```python
from build123d import *

# Parameters (mm, degrees)
SKETCH1_W               = 52
SKETCH1_H               = 25
BOSS_EXTRUDE1_DEPTH     = 24.18
SKETCH4_W               = 48
SKETCH4_H               = 21.11598097
CUT_EXTRUDE1_DEPTH      = 25
SKETCH6_R               = 1
SKETCH6_R_2             = 1.5
CUT_EXTRUDE5_DEPTH      = 24.18
SKETCH8_W               = 25
SKETCH8_H               = 5
BOSS_EXTRUDE2_DEPTH     = 15
SKETCH9_R               = 1.5
CUT_EXTRUDE7_DEPTH      = 5
MIRROR4_COPY_1_SKETCH_R = 1.5
MIRROR4_COPY_1_DEPTH    = 5


with BuildPart() as part:
    # Sketch1 → Boss-Extrude1 (new body)
    with BuildSketch(Plane(origin=(0, 0, 0), x_dir=(1, 0, 0), z_dir=(0, 1, 0))):
        Rectangle(SKETCH1_W, SKETCH1_H)
    extrude(amount=BOSS_EXTRUDE1_DEPTH)

    # Sketch4 → Cut-Extrude1 (cut)
    with BuildSketch(Plane.XY.offset(12.5)):
        with Locations((0, 15.557990485)):
            Rectangle(SKETCH4_W, SKETCH4_H)
    extrude(amount=-CUT_EXTRUDE1_DEPTH, mode=Mode.SUBTRACT)

    # Sketch6 → Cut-Extrude5 (cut)
    with BuildSketch(Plane.XZ):
        with Locations(Location((-7.75, 0, 0), (0, 0, 270))):
            Circle(SKETCH6_R)
        with Locations(Location((-20, 0, 0), (0, 0, 270))):
            Circle(SKETCH6_R_2)
        with Locations(Location((7.75, 0, 0), (0, 0, 270))):
            Circle(SKETCH6_R)
        with Locations(Location((20, 0, 0), (0, 0, 270))):
            Circle(SKETCH6_R_2)
    extrude(amount=-CUT_EXTRUDE5_DEPTH, mode=Mode.SUBTRACT)

    # Sketch8 → Boss-Extrude2 (add)
    with BuildSketch(Plane(origin=(26, 0, 0), x_dir=(0, 0, -1), z_dir=(1, 0, 0))):
        with Locations((0, 21.68)):
            Rectangle(SKETCH8_W, SKETCH8_H)
    boss_extrude2 = extrude(amount=BOSS_EXTRUDE2_DEPTH)

    # Sketch9 → Cut-Extrude7 (cut)
    with BuildSketch(Plane(origin=(0, 24.18, 0), x_dir=(1, 0, 0), z_dir=(0, 1, 0))):
        with Locations(Location((33, 6.5, 0), (0, 0, 270))):
            Circle(SKETCH9_R)
    cut_extrude7 = extrude(amount=-CUT_EXTRUDE7_DEPTH, mode=Mode.SUBTRACT)

    # Mirror3: Cut-Extrude7 across plane
    add(cut_extrude7.mirror(Plane.XY), mode=Mode.SUBTRACT)

    # Mirror4: Boss-Extrude2, Cut-Extrude7 across plane
    add(boss_extrude2.mirror(Plane(origin=(0, 0, 0), x_dir=(0, 0, 1), z_dir=(1, 0, 0))))
    add(cut_extrude7.mirror(Plane(origin=(0, 0, 0), x_dir=(0, 0, 1), z_dir=(1, 0, 0))), mode=Mode.SUBTRACT)

    # Mirror4 copy 1 sketch → Mirror4 copy 1 (cut)
    with BuildSketch(Plane(origin=(0, 24.18, 0), x_dir=(-1, 0, 0), z_dir=(0, 1, 0))):
        with Locations(Location((33, 6.5, 0), (0, 0, 270))):
            Circle(MIRROR4_COPY_1_SKETCH_R)
    extrude(amount=-MIRROR4_COPY_1_DEPTH, mode=Mode.SUBTRACT)


solid = part.part
```
Here's how the part is built. I have some questions about the finished solid (model axes, mm). A direction names the side the tool comes from. Round coordinates to 2 decimals unless told otherwise and drop trailing zeros. Order: outer loops, then holes, each group sorted by start corner. A loop starts at its lowest first (then second) coordinate and runs counter-clockwise, first axis right, second up. Notation, with made-up numbers: M 55.25,-30.5 L 75.25,-30.5 A24 ccw 75.25,7.5 Z; hole C 7,43 d10. An arc over 180 degrees is marked long. Use CSV: the item, a comma, the result in double quotes.
1) I want a section at B-B (y = 21.5). List the corners of the cut face in (x, z) for me.
Taken from the geometry:
outline,"M -41,-12.5 L -24,-12.5 L -24,12.5 L -41,12.5 Z; M 24,-12.5 L 41,-12.5 L 41,12.5 L 24,12.5 Z; hole C -33,-6.5 d3; hole C -33,6.5 d3; hole C 33,-6.5 d3; hole C 33,6.5 d3"
2) On a 3-axis mill with a long thin cutter (end or side, diameter ignored), from which of +Z, -Z, +X, -X, +Y, -Y can I reach the whole of each face in a straight line? I mean faces 1 (the cylindrical face through (-31.536, 21.715, -6.825)), 2 (the flat face through (26, 9, 0)), 3 (the flat face through (41, 22, 0)), 4 (the flat face through (24, 14, 0)), 5 (the flat face through (-26, 9, 0)). Say none if no direction works.
Taken from the geometry:
face 1,"+Y, -Y"
face 2,"+Z, -Z, +X, -Y"
face 3,"+Z, -Z, +X, +Y, -Y"
face 4,"+Z, -Z, +Y"
face 5,"+Z, -Z, -X, -Y"
3) I want a section at A-A (x = 20). List the corners of the cut face in (y, z) for me.
Taken from the geometry:
outline,"M 0,-12.5 L 5,-12.5 L 5,-1.5 L 0,-1.5 Z; M 0,1.5 L 5,1.5 L 5,12.5 L 0,12.5 Z"
4) I want a section at D-D (y = 8). List the corners of the cut face in (x, z) for me.
Taken from the geometry:
outline,"M -26,-12.5 L -24,-12.5 L -24,12.5 L -26,12.5 Z; M 24,-12.5 L 26,-12.5 L 26,12.5 L 24,12.5 Z"
5) I'm going to push flat-ended pins straight in: P1, Ø4, axis at y = 14.5, z = 0.5, coming from the +X side; P2, Ø2.5, axis at x = 33, z = -6.5, coming from the -Y side; P3, Ø9.5, axis at y = 12.5, z = 4, coming from the -X side; P4, Ø12, axis at x = 34, z = 0.5, coming from the -Y side. Where does each tip first touch, or does it pass through?
Taken from the geometry:
P1,"x = 26"
P2,"through"
P3,"x = -26"
P4,"y = 19.18"
6) If we mould it in two halves opening along Z, with no side actions, what happens to faces 6 (the flat face through (-32, 24.18, 0)), 7 (the flat face through (-3, 4, 12.5)), 8 (the cylindrical face through (21.265, 2.465, -0.806)), 9 (the flat face through (-3, 4, -12.5))? For each: pulls with the +Z half, pulls with the -Z half, needs draft (parallel to the pull), parting line crosses it, or undercut.
Taken from the geometry:
face 6,"needs draft"
face 7,"pulls with the +Z half"
face 8,"undercut"
face 9,"pulls with the -Z half"
7) I want a section at C-C (z = 6.5). List the corners of the cut face in (x, y) for me, then the cut area to 3 significant figures.
Taken from the geometry:
outline,"M -41,19.18 L -34.5,19.18 L -34.5,24.18 L -41,24.18 Z; M -31.5,19.18 L -26,19.18 L -26,0 L 26,0 L 26,19.18 L 31.5,19.18 L 31.5,24.18 L 24,24.18 L 24,5 L -24,5 L -24,24.18 L -31.5,24.18 Z; M 34.5,19.18 L 41,19.18 L 41,24.18 L 34.5,24.18 Z"
area,"457 mm^2"
8) I need wall thicknesses on line 1 along X through (y, z) = (20.35, -6.5); line 2 along X through (y, z) = (3, 0); line 3 along X through (y, z) = (15.25, -1). Which ranges of each line are inside material? Lowest first, please. Write a range as [from, to].
Taken from the geometry:
line 1,"[-41, -34.5], [-31.5, -24], [24, 31.5], [34.5, 41]"
line 2,"[-26, -21.5], [-18.5, -8.75], [-6.75, 6.75], [8.75, 18.5], [21.5, 26]"
line 3,"[-26, -24], [24, 26]"
